Autodesk Inventor part; units mm, degrees
ref_plane "YZ Plane" through (0, 0, 0) normal (1, 0, 0) x (0, 1, 0)
ref_plane "XZ Plane" through (0, 0, 0) normal (0, 1, 0) x (-1, 0, 0)
ref_plane "XY Plane" through (0, 0, 0) normal (0, 0, 1) x (1, 0, 0)
sketch "Sketch1" plane through (0, 0, 0) normal (0, 1, 0) x (-1, 0, 0)
  line L0 (-89, 127) -> (89, 127)
  line L1 (89, 127) -> (89, -127)
  line L2 (89, -127) -> (-89, -127)
  line L3 (-89, -127) -> (-89, 127)
  line L4 (-89, 127) -> (89, -127) construction
  line L5 (89, 127) -> (-89, -127) construction
  line L6 (90, 128) -> (-90, 128)
  line L7 (-90, 128) -> (-90, -128)
  line L8 (-90, -128) -> (90, -128)
  line L9 (90, -128) -> (90, 128)
  point P0 (0, 0)
  dimension "d0" = 178
  dimension "d1" = 254
  dimension "d2" = 1
extrude "Extrusion1" add sketch "Sketch1" along normal blind 101.6
sketch "Sketch3" plane through (0, 0, 0) normal (0, -1, 0) x (1, 0, 0)
  line L0 (90, 128) -> (90, -128)
  line L1 (90, -128) -> (-90, -128)
  line L2 (90, 128) -> (90, -128)
  line L3 (90, -128) -> (115, -128)
  line L4 (115, -128) -> (115, 128)
  line L5 (115, 128) -> (90, 128)
  line L6 (90, -128) -> (-90, -128)
  line L7 (-90, -128) -> (-90, -153)
  line L8 (-90, -153) -> (90, -153)
  line L9 (90, -153) -> (90, -128)
  line L10 (-90, 128) -> (90, 128)
  line L11 (-90, -128) -> (-90, 128)
  line L12 (-90, 128) -> (-115, 128)
  line L13 (-115, 128) -> (-115, -128)
  line L14 (-115, -128) -> (-90, -128)
  line L15 (-90, 128) -> (90, 128)
  line L16 (90, 128) -> (90, 153)
  line L17 (90, 153) -> (-90, 153)
  line L18 (-90, 153) -> (-90, 128)
  point P0 (0, 0)
  dimension "d11" = 25
  dimension "d12" = 25
  dimension "d13" = 25
  dimension "d14" = 25
extrude "Extrusion3" add sketch "Sketch3" against normal blind 0.8 contours L5 L4 L3 L0 | L10 L18 L17 L16 | L9 L8 L7 L1 | L11 L14 L13 L12
sketch "Sketch4" plane through (0, 0.8, 0) normal (0, 1, 0) x (1, 0, 0)
  line L0 (101.5, 139.5) -> (-101.5, 139.5) construction
  line L1 (-101.5, 139.5) -> (-101.5, -139.5) construction
  line L2 (-101.5, -139.5) -> (101.5, -139.5) construction
  line L3 (101.5, -139.5) -> (101.5, 139.5) construction
  line L4 (101.5, 139.5) -> (-101.5, -139.5) construction
  line L5 (-101.5, 139.5) -> (101.5, -139.5) construction
  line L6 (0, 0) -> (0, -60) construction
  line L7 (0, 0) -> (60, 0) construction
  point P0 (-101.5, 0)
  point P1 (101.5, 0)
  point P2 (101.5, 104.625)
  point P3 (101.5, 69.75)
  point P4 (101.5, 34.875)
  point P5 (101.5, 0)
  point P6 (101.5, -34.875)
  point P7 (101.5, -69.75)
  point P8 (101.5, -104.625)
  point P9 (67.6667, 139.5)
  point P10 (33.8333, 139.5)
  point P11 (0, 139.5)
  point P12 (-33.8333, 139.5)
  point P13 (-67.6667, 139.5)
  point P14 (-101.5, 139.5)
  point P15 (67.6667, -139.5)
  point P16 (33.8333, -139.5)
  point P17 (0, -139.5)
  point P18 (-33.8333, -139.5)
  point P19 (-67.6667, -139.5)
  point P20 (-101.5, -139.5)
  point P21 (-101.5, 104.625)
  point P22 (-101.5, 69.75)
  point P23 (-101.5, 34.875)
  point P24 (-101.5, 0)
  point P25 (-101.5, -34.875)
  point P26 (-101.5, -69.75)
  point P27 (-101.5, -104.625)
  dimension "d18" = 203
  dimension "d19" = 279
  dimension "d21" = 60
  dimension "d22" = 90
  dimension "d63" = 34.875
  dimension "d70" = 33.8333
  dimension "d77" = 33.8333
  dimension "d84" = 34.875
hole "Hole1" at (101.5, 0.8, -139.5) at (101.5, 0.8, -104.625) at (101.5, 0.8, -34.875) at (101.5, 0.8, 34.875) at (101.5, 0.8, 104.625) at (101.5, 0.8, 139.5) at (67.6667, 0.8, -139.5) at (0, 0.8, -139.5) at (-67.6667, 0.8, -139.5) at (-101.5, 0.8, -139.5) at (67.6667, 0.8, 139.5) at (0, 0.8, 139.5) at (-67.6667, 0.8, 139.5) at (-101.5, 0.8, 139.5) at (-101.5, 0.8, -104.625) at (-101.5, 0.8, -34.875) at (-101.5, 0.8, 34.875) at (-101.5, 0.8, 104.625) direction (0, -1, 0) diameter 6 end through all
sketch "Sketch9" plane through (90, 0.8, 128) normal (1, 0, 0) x (0, 0, -1)
  line L0 (0, 100.8) -> (14.1421, 114.9421)
  line L1 (0, 100.8) -> (20, 100.8) construction
  line L2 (14.5421, 114.5421) -> (0.8, 100.8)
  line L3 (14.1421, 114.9421) -> (14.5421, 114.5421)
  line L4 (256, 0) -> (256, 100.8)
  line L5 (256, 100.8) -> (241.8579, 114.9421)
  line L6 (256, 100.8) -> (276, 100.8) construction
  line L7 (0, 100.8) -> (256, 100.8)
  line L8 (229, 100.8) -> (256, 100.8)
  line L9 (256, 100.8) -> (0, 100.8)
  line L10 (0, 100.8) -> (0.8, 100.8)
  line L11 (241.2922, 114.3765) -> (254.8686, 100.8)
  line L12 (241.8579, 114.9421) -> (241.2922, 114.3765)
  point P0 (128, -0.8)
  dimension "d51" = 20
  dimension "d52" = 45
  dimension "d53" = 20
  dimension "d54" = 135
  dimension "d89" = 0.8
extrude "Extrusion8" add sketch "Sketch9" against normal up to surface (180 mm away)
properties part number "chimneyHousing"
Here's how the part is built. I have some questions about the finished solid (model axes, mm). A direction names the side the tool comes from. Round coordinates to 2 decimals unless told otherwise and drop trailing zeros. Loops run counter-clockwise (first coordinate to the right, second up) from the corner with the lowest first, then second, coordinate; pieces in that order, holes last. Notation, with made-up numbers: M 50,-4.75 L 104,-4.75 A19 cw 104,10.25 Z; hole C 43,-40 d5. An arc over 180 degrees is marked long. Write each question's results on one line, items separated by ' | '. Start each with the question number.
(1) On a 3-axis mill with a long thin cutter (end or side, diameter ignored), from which of +Z, -Z, +X, -X, +Y, -Y can I reach the whole of each face in a straight line? I mean faces 1 (the flat face through (-1, 50, -127)), 2 (the flat face through (90, 45, 2)), 3 (the cylindrical face through (104.429, 0.394, -105.275)). Say none if no direction works.
(2) I want a section at B-B (x = -27). Please give me the cut outline in (y, z), then the cut area to 3 significant figures.
(3) Thinking about a two-plate mould opening in X: for faces 4 (the flat face through (-90, 45, -2)), 5 (the cylindrical face through (-66.518, 0.394, 142.271)), 6 (the flat face through (-94, 0, 1)), which applies, pulls with the +X half, pulls with the -X half, needs draft (parallel to the pull), parting line crosses it, or undercut?
(4) If I drill on probe 1 along Z at (x, y) = (-101.5, 0.55) (3 decimals); probe 2 along X at (y, z) = (8, 33); probe 3 along Z at (x, y) = (-53.5, 34.5), over which ranges is the centre line in solid material (lowest first)? Write a range as from..to.
(5) I want a section at A-A (z = -98). Please give me the cut outline in (x, y).
(6) Will these pins go through, and if not, where does the flat tip stop? P1, Ø12, axis at x = -78.5, z = -103.5, coming from the -Y side; P2, Ø7.5, axis at x = 104.5, z = 3.5, coming from the +Y side; P3, Ø8, axis at x = 27, y = 37.5, coming from the +Z side; P4, Ø6, axis at y = 18.5, z = -101, coming from the +X side.
(7) I want a section at C-C (y = 23). Please give me the cut outline in (x, z).
Solved:
1) face 1: -Y | face 2: +Z, -Z, +X, +Y | face 3: +Y, -Y
2) outline: M 0,-153 L 0.8,-153 L 0.8,-128 L 101.6,-128 L 115.74,-113.86 L 115.18,-113.29 L 101.6,-126.87 L 101.6,-127 L 0,-127 Z; M 0,127 L 101.6,127 L 101.6,127.2 L 115.34,113.46 L 115.74,113.86 L 101.6,128 L 0.8,128 L 0.8,153 L 0,153 Z | area: 270 mm²
3) face 4: pulls with the -X half | face 5: undercut | face 6: needs draft
4) probe 1: z = -128..-107.625, -101.625..-37.875, -31.875..31.875, 37.875..101.625, 107.625..128 | probe 2: x = -90..-89, 89..90 | probe 3: z = -128..-127, 127..128
5) outline: M -115,0 L -89,0 L -89,101.6 L -90,101.6 L -90,0.8 L -115,0.8 Z; M 89,0 L 115,0 L 115,0.8 L 90,0.8 L 90,101.6 L 89,101.6 Z
6) P1: passes through | P2: stops at y = 0.8 | P3: stops at z = 128 | P4: stops at x = 90
7) outline: M -90,-128 L 90,-128 L 90,128 L -90,128 Z; hole M -89,-127 L 89,-127 L 89,127 L -89,127 Z
